Autodesk Fusion 360 part; units mm, degrees
sketch "Sketch1" plane through (0, 0, 0) normal (0, 0, 1) x (1, 0, 0)
  line L0 (-20.375, 17.825) -> (20.375, 17.825)
  line L1 (20.375, 17.825) -> (20.375, -17.825)
  line L2 (20.375, -17.825) -> (-20.375, -17.825)
  line L3 (-20.375, -17.825) -> (-20.375, 17.825)
  line L4 (-20.375, 17.825) -> (20.375, -17.825) construction
  line L5 (20.375, 17.825) -> (-20.375, -17.825) construction
  dimension "d1" = 40.75
  dimension "d2" = 35.65
extrude "Extrude1" add sketch "Sketch1" along normal blind 20
sketch "Sketch2" plane through (20.375, 0, 0) normal (1, 0, 0) x (0, 1, 0)
  line L0 (-17.825, 0) -> (17.825, 0)
  line L1 (17.825, 0) -> (17.825, 20)
  line L2 (17.825, 20) -> (-17.825, 20)
  line L3 (-17.825, 20) -> (-17.825, 0)
  line L4 (17.825, 20) -> (11.625, 20)
  line L5 (11.625, 20) -> (9.125, 20)
  line L6 (9.125, 20) -> (9.125, 0)
  line L7 (9.125, 0) -> (11.625, 0)
  line L8 (11.625, 0) -> (11.625, 20)
  dimension "d5" = 6.2
  dimension "d6" = 2.5
extrude "Extrude2" add sketch "Sketch2" along normal blind 7 contours L0 L2 L5 L6 L7 L8
sketch "Sketch3" plane through (20.375, 0, 0) normal (1, 0, 0) x (0, 1, 0)
  line L0 (11.625, 20) -> (11.625, 0)
  line L1 (11.625, 0) -> (17.825, 0)
  line L2 (17.825, 0) -> (17.825, 20)
  line L3 (17.825, 20) -> (11.625, 20)
  line L4 (11.625, 20) -> (11.625, 11.25)
  line L5 (11.625, 0) -> (11.625, 8.75)
  line L6 (17.825, 10) -> (13.575, 10)
  line L7 (11.625, 11.25) -> (13.575, 11.25)
  line L8 (13.575, 11.25) -> (13.575, 10)
  line L9 (13.575, 10) -> (11.625, 10)
  line L10 (11.625, 10) -> (11.625, 11.25)
  line L11 (13.575, 10) -> (11.625, 10)
  line L12 (11.625, 10) -> (11.625, 8.75)
  line L13 (11.625, 8.75) -> (13.575, 8.75)
  line L14 (13.575, 8.75) -> (13.575, 10)
  dimension "d9" = 8.75
  dimension "d10" = 8.75
  dimension "d11" = 4.25
extrude "Extrude3" add sketch "Sketch3" along normal blind 7 contours L0 L7 L8 L9 L10 L11 | L0 L9 L11 L12 L13 L14
extrude "Extrude4" add 1 faces at (27.375, 9.9583, 9.5833) along direction (-1, 0, 0) blind 55
sketch "Sketch4" plane through (20.375, 0, 0) normal (1, 0, 0) x (0, 1, 0)
  line L0 (9.125, 0) -> (9.125, 20)
  line L1 (9.125, 20) -> (-17.825, 20)
  line L2 (-17.825, 20) -> (-17.825, 0)
  line L3 (-17.825, 0) -> (9.125, 0)
sketch "Sketch5" plane through (20.375, 0, 0) normal (1, 0, 0) x (0, 1, 0)
  line L0 (-15, 20) -> (-15, 13.7)
  line L1 (-17.8217, 13.7) -> (-14.9217, 13.7)
  line L2 (-14.9217, 0) -> (-14.9217, 6.3)
  line L3 (-14.9217, 6.3) -> (-10.6217, 6.3)
  line L4 (-10.6217, 6.3) -> (-10.6217, 13.7)
  line L5 (-10.6217, 13.7) -> (-14.9217, 13.7)
  line L6 (-14.9217, 13.7) -> (-14.9217, 6.3)
  dimension "d16" = 6.3
  dimension "d17" = 2.9
  dimension "d18" = 6.3
  dimension "d19" = 4.3
extrude "Extrude5" add sketch "Sketch5" along normal blind 5.9
sketch "Sketch6" plane through (0, 17.825, 0) normal (0, 1, 0) x (-1, 0, 0)
  line L0 (-20.375, 0) -> (20.375, 0)
  line L1 (20.375, 0) -> (20.375, 20)
  line L2 (20.375, 20) -> (-20.375, 20)
  line L3 (-20.375, 20) -> (-20.375, 0)
  line L4 (-20.375, 4.9972) -> (-14.025, 4.9972)
  line L5 (-14, 0) -> (-14, 0.75)
  line L6 (-14, 20) -> (-14, 19.25)
  line L7 (-14, 0.75) -> (6, 0.75)
  line L8 (6, 0.75) -> (6, 19.25)
  line L9 (6, 19.25) -> (-14, 19.25)
  line L10 (-14, 19.25) -> (-14, 0.75)
  circle A0 centre (10.3, 10) radius 10
  dimension "d22" = 6.35
  dimension "d23" = 0.75
  dimension "d24" = 0.75
  dimension "d25" = 20
  dimension "d26" = 18.5
extrude "Extrude6" add sketch "Sketch6" along normal blind 1.75 contours L8 A0 | L7 L8 L9 L10 A0 | L8 A0
sketch "Sketch7" plane through (0, 19.575, 0) normal (0, 1, 0) x (-1, 0, 0)
  arc A0 (6, 0.9717) -> (6, 19.0283) centre (10.3, 10) ccw
  line L0 (6, 19.0283) -> (6, 19.25)
  line L1 (6, 19.25) -> (-14, 19.25)
  line L2 (-14, 19.25) -> (-14, 0.75)
  line L3 (-14, 0.75) -> (6, 0.75)
  line L4 (6, 0.75) -> (6, 0.9717)
  circle A1 centre (10.3, 10) radius 6.45
  circle A2 centre (10.3, 10) radius 5.6
  circle A3 centre (10.3, 10) radius 2.9
  dimension "d29" = 12.9
  dimension "d30" = 11.2
  dimension "d31" = 5.8
extrude "Extrude7" add sketch "Sketch7" along normal blind 1.4 contours A1
extrude "Extrude8" add 1 faces at (-12.8422, 19.575, 11.496) along direction (0, 1, 0) blind 2.1
sketch "Sketch8" plane through (0, 21.675, 0) normal (0, 1, 0) x (-1, 0, 0)
  circle A0 centre (10.3, 10) radius 5.6
sketch "Sketch9" plane through (0, 21.675, 0) normal (0, 1, 0) x (-1, 0, 0)
  curve A0
  circle A1 centre (10.3, 10) radius 2.9063
  circle A2 centre (10.3, 10) radius 5.6
  circle A3 centre (10.3, 10) radius 2.9063
  point P0 (10.3, 10)
extrude "Extrude9" add sketch "Sketch9" along normal blind 3.5 contours A1 A3
sketch "Sketch10" plane through (0, 17.825, 0) normal (0, 1, 0) x (-1, 0, 0)
  arc A0 (10.3, 20) -> (6, 19.0283) centre (10.3, 10) ccw
  line L0 (10.3, 20) -> (-20.375, 20)
  line L1 (-20.375, 20) -> (-20.375, 0)
  line L2 (-20.375, 0) -> (10.3, 0)
  arc A1 (6, 0.9717) -> (10.3, 0) centre (10.3, 10) ccw
  line L3 (6, 0.9717) -> (6, 0.75)
  line L4 (6, 0.75) -> (-14, 0.75)
  line L5 (-14, 0.75) -> (-14, 19.25)
  line L6 (-14, 19.25) -> (6, 19.25)
  line L7 (6, 19.25) -> (6, 19.0283)
  line L8 (-14, 14.875) -> (-14, 5.125)
  circle A2 centre (-12.2062, 10.0187) radius 5.0718
  point P0 (-14, 10)
  dimension "d38" = 9.75
extrude "Extrude10" add sketch "Sketch10" along normal blind 1.75 contours L5 L8 A2 picked at (-10.7739, 9.0841)
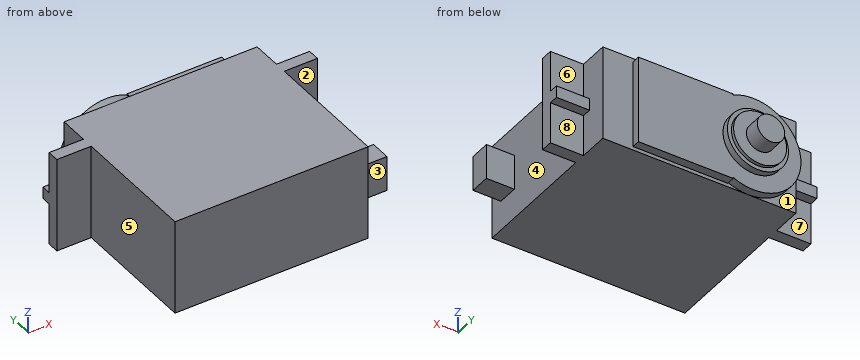
Read the model definition and answer for the solid it produces. Units are mm, in the model's axes. Face numbers are marked on the shaded views. A direction names the side the tool comes from. Give positions to 0.01 mm unless a question says otherwise; leave off trailing zeros. Write each loop counter-clockwise with the first axis right and the second up, starting at its lowest first coordinate (ties: lowest second). Pieces come first, ordered by that corner, then holes. Notation, with made-up numbers: (24.5, 25) - (65.5, 25) arc R25 ccw to (65.5, 37) - close; hole circle Ø4 at (57, 55.25). An arc over 180 degrees is marked (long way). Use CSV: the item, a comma, the result in double quotes. Start each with the question number.
(1) Find section B-B (x = 3.5). Give the vertices of the cut face in (y, z) (3 decimals), plus the area to 3 significant figures.
(2) For the marked faces 5, 6, 7 and 8, determine the directions among +Z, -Z, +X, -X, +Y, -Y from which every point of the face is accessible in a straight line to the end or side of a thin tool.
(3) Determine the mould class of the marked faces 1, 2, 3 and 4 for opening direction Y: +Y half, -Y half, draft (parallel to the pull), parting line (faces both ways), or undercut.
(4) Find section D-D (z = 14.5). Give the vertices of the cut face in (x, y) (3 decimals).
(5) Find section A-A (x = 22). Give the vertices of the cut face in (y, z) (3 decimals).
(6) Find section C-C (y = 2.5). Give the vertices of the cut face in (x, z) (3 decimals), plus the area to 3 significant figures.
(7) Given P1, Ø3, axis at x = 22.5, z = 9.5, coming from the +Y side (3 decimals); P2, Ø3.5, axis at x = 24.5, y = -13, coming from the +Z side; P3, Ø2, axis at y = 13.5, z = 16, coming from the +X side (3 decimals), each flat-ended and moving along its own axis, determine where each tip first touches the part or whether it passes through.
(8) Consider line 1 along Y through (x, z) = (21.5, 13) (3 decimals); line 2 along Y through (x, z) = (22, 9.25) (3 decimals); line 3 along Y through (x, z) = (18.5, 1.5) (3 decimals). Determine where each line is inside the solid, lowest interval first.
Findings below:
1,outline,"(-17.825, 0) - (17.825, 0) - (17.825, 0.75) - (19.575, 0.75) - (19.575, 19.25) - (17.825, 19.25) - (17.825, 20) - (-17.825, 20) - close"
1,area,"745 mm2"
2,face 5,"+Z, -Z, -X, -Y"
2,face 6,"+Z, +X, +Y"
2,face 7,"-Z, -X, +Y"
2,face 8,"-Z, +X, +Y"
3,face 1,"+Y half"
3,face 2,"undercut"
3,face 3,"-Y half"
3,face 4,"undercut"
4,outline,"(-27.625, 9.125) - (-20.375, 9.125) - (-20.375, -17.825) - (20.375, -17.825) - (20.375, 9.125) - (27.375, 9.125) - (27.375, 11.625) - (20.375, 11.625) - (20.375, 17.825) - (14, 17.825) - (14, 19.575) - (-5.679, 19.575) - (-5.679, 20.975) - (-6.967, 20.975) - (-6.967, 21.675) - (-13.633, 21.675) - (-13.633, 20.975) - (-14.921, 20.975) - (-14.921, 19.575) - (-19.23, 19.575) - (-19.23, 17.825) - (-20.375, 17.825) - (-20.375, 11.625) - (-27.625, 11.625) - close"
5,outline,"(-14.922, 6.3) - (-10.622, 6.3) - (-10.622, 13.7) - (-14.922, 13.7) - close; (9.125, 0) - (11.625, 0) - (11.625, 8.75) - (13.575, 8.75) - (13.575, 11.25) - (11.625, 11.25) - (11.625, 20) - (9.125, 20) - close"
6,outline,"(-20.375, 0) - (20.375, 0) - (20.375, 20) - (-20.375, 20) - close"
6,area,"815 mm2"
7,P1,"y = 13.575"
7,P2,"z = 13.7"
7,P3,"x = 20.375"
8,line 1,"-14.922 to -10.622, 9.125 to 11.625"
8,line 2,"-14.922 to -10.622, 9.125 to 13.575"
8,line 3,"-17.825 to 17.825"
